Read the model definition and answer for the solid it produces. Units are mm, in the model's axes. A direction names the side the tool comes from. Coordinates: 2 decimals unless noted, no trailing zeros. Loops run counter-clockwise (first coordinate to the right, second up) from the corner with the lowest first, then second, coordinate; pieces in that order, holes last. Notation, with made-up numbers: (13, 88.5) -> (26, 88.5) arc R13 cw to (26, 94.5) -> close; hole circle Ø9 at (-17.75, -12). An arc over 180 degrees is marked (long way). Answer in a Markdown table with one row per item.
```python
from build123d import *

# Parameters (mm, degrees)
BOSS_EXTRUDE1_DEPTH = 24
SKETCH2_R           = 5
BOSS_EXTRUDE2_DEPTH = 16
FILLET1_R           = 2
SKETCH4_W           = 5.41
SKETCH4_H           = 3.8
CUT_EXTRUDE1_DEPTH  = 20


with BuildPart() as part:
    # Sketch1 → Boss-Extrude1 (new body)
    with BuildSketch(Plane(origin=(0, 0, 0), x_dir=(0, 0, -1), z_dir=(1, 0, 0))):
        with BuildLine():
            Line((2.314035395, 32.242240005), (10.473918124, 39.089194593))
            Line((10.473918124, 39.089194593), (14.117106565, 29.079616616))
            ThreePointArc((14.117106565, 29.079616616), (15.7, 27.193197679), (18.12513344, 26.765581222))
            Line((18.12513344, 26.765581222), (28.615276469, 28.615276469))
            Line((28.615276469, 28.615276469), (26.765581222, 18.12513344))
            ThreePointArc((26.765581222, 18.12513344), (27.193197679, 15.7), (29.079616616, 14.117106565))
            Line((29.079616616, 14.117106565), (39.089194593, 10.473918124))
            Line((39.089194593, 10.473918124), (32.242240005, 2.314035395))
            ThreePointArc((32.242240005, 2.314035395), (31.4, 0), (32.242240005, -2.314035395))
            Line((32.242240005, -2.314035395), (39.089194593, -10.473918124))
            Line((39.089194593, -10.473918124), (29.079616616, -14.117106565))
            ThreePointArc((29.079616616, -14.117106565), (27.193197679, -15.7), (26.765581222, -18.12513344))
            Line((26.765581222, -18.12513344), (28.615276469, -28.615276469))
            Line((28.615276469, -28.615276469), (18.12513344, -26.765581222))
            ThreePointArc((18.12513344, -26.765581222), (15.7, -27.193197679), (14.117106565, -29.079616616))
            Line((14.117106565, -29.079616616), (10.473918124, -39.089194593))
            Line((10.473918124, -39.089194593), (2.314035395, -32.242240005))
            ThreePointArc((2.314035395, -32.242240005), (0, -31.4), (-2.314035395, -32.242240005))
            Line((-2.314035395, -32.242240005), (-10.473918124, -39.089194593))
            Line((-10.473918124, -39.089194593), (-14.117106565, -29.079616616))
            ThreePointArc((-14.117106565, -29.079616616), (-15.7, -27.193197679), (-18.12513344, -26.765581222))
            Line((-18.12513344, -26.765581222), (-28.615276469, -28.615276469))
            Line((-28.615276469, -28.615276469), (-26.765581222, -18.12513344))
            ThreePointArc((-26.765581222, -18.12513344), (-27.193197679, -15.7), (-29.079616616, -14.117106565))
            Line((-29.079616616, -14.117106565), (-39.089194593, -10.473918124))
            Line((-39.089194593, -10.473918124), (-32.242240005, -2.314035395))
            ThreePointArc((-32.242240005, -2.314035395), (-31.4, 0), (-32.242240005, 2.314035395))
            Line((-32.242240005, 2.314035395), (-39.089194593, 10.473918124))
            Line((-39.089194593, 10.473918124), (-29.079616616, 14.117106565))
            ThreePointArc((-29.079616616, 14.117106565), (-27.193197679, 15.7), (-26.765581222, 18.12513344))
            Line((-26.765581222, 18.12513344), (-28.615276469, 28.615276469))
            Line((-28.615276469, 28.615276469), (-18.12513344, 26.765581222))
            ThreePointArc((-18.12513344, 26.765581222), (-15.7, 27.193197679), (-14.117106565, 29.079616616))
            Line((-14.117106565, 29.079616616), (-10.473918124, 39.089194593))
            Line((-10.473918124, 39.089194593), (-2.314035395, 32.242240005))
            ThreePointArc((-2.314035395, 32.242240005), (0, 31.4), (2.314035395, 32.242240005))
        make_face()
    extrude(amount=BOSS_EXTRUDE1_DEPTH)

    # Sketch2 → Boss-Extrude2 (add)
    with BuildSketch(Plane(origin=(24, 0, 0), x_dir=(0, 0, -1), z_dir=(1, 0, 0))):
        Circle(SKETCH2_R)
    extrude(amount=BOSS_EXTRUDE2_DEPTH)

    # Fillet1
    fillet1_edges = [part.edges().sort_by_distance(p)[0] for p in [
        (24, 0, 5),
    ]]
    fillet(fillet1_edges, radius=FILLET1_R)

    # Sketch4 → Cut-Extrude1 (cut)
    with BuildSketch(Plane(origin=(40, 0, 0), x_dir=(0, 0, -1), z_dir=(1, 0, 0))):
        Rectangle(SKETCH4_W, SKETCH4_H)
    extrude(amount=-CUT_EXTRUDE1_DEPTH, mode=Mode.SUBTRACT)


solid = part.part
```
1. Given pin 1 Ø1.9 at (x, y) = (26, -1) entering from +Z; pin 2 Ø3 at (x, y) = (9.5, -4.5) entering from -Z; pin 3 Ø1.1 at (x, y) = (34.5, -1) entering from -Z; pin 4 Ø5 at (y, z) = (-17.5, -30) entering from -X, each flat-ended and moving along its own axis, determine where each tip first touches the part or whether it passes through.
A:
| item | result |
|---|---|
| pin 1 | stops at z = 5.17 |
| pin 2 | stops at z = -35.34 |
| pin 3 | stops at z = -4.98 |
| pin 4 | passes through |
2. The mould has two halves that part along Z. Classify faces 5 (the flat face through (11.832, 6.451, -35.714)), 6 (the cylindrical face through (11.832, -27.176, -15.731)), 7 (the flat face through (11.832, -23.444, 27.703)): pulls with the +Z half, pulls with the -Z half, needs draft (parallel to the pull), parting line crosses it, or undercut.
A:
| item | result |
|---|---|
| face 5 | pulls with the -Z half |
| face 6 | undercut |
| face 7 | pulls with the +Z half |
3. A tool of negligible diameter and unlimited length cuts with its end or side. For faces 1 (the flat face through (11.832, 27.703, 23.444)), 2 (the flat face through (20, 0, 0)), 3 (the flat face through (11.83, 23.3, 27.68)), 4 (the flat face through (11.83, -23.3, -27.68)), from which of +Z, -Z, +X, -X, +Y, -Y can it reach the whole face along a straight path? Write none if from no direction.
A:
| item | result |
|---|---|
| face 1 | +X, -X, +Y |
| face 2 | +X |
| face 3 | +Z, +X, -X |
| face 4 | -Z, +X, -X |
4. Find the intervals of material crossed by probe 1 along X at (y, z) = (-1.5, 1); probe 2 along X at (y, z) = (-32, -3); probe 3 along Y at (x, z) = (23, 17), in increasing order.
A:
| item | result |
|---|---|
| probe 1 | x = 0 to 20 |
| probe 2 | x = 0 to 24 |
| probe 3 | y = -26.75 to 26.75 |
5. A cutting plane is placed at A-A on y = 0. Give the vertices of the cut face in (x, z) (3 decimals), and give its area (3 significant figures).
A:
| item | result |
|---|---|
| outline | (0, -31.4) -> (24, -31.4) -> (24, -7) arc R2 cw to (26, -5) -> (40, -5) -> (40, -2.705) -> (20, -2.705) -> (20, 2.705) -> (40, 2.705) -> (40, 5) -> (26, 5) arc R2 cw to (24, 7) -> (24, 31.4) -> (0, 31.4) -> close |
| area | 1,560 mm2 |
6. A cutting plane is placed at B-B on z = 0. Give the vertices of the cut face in (x, y), and give its area (3 significant figures).
A:
| item | result |
|---|---|
| outline | (0, -31.4) -> (24, -31.4) -> (24, -7) arc R2 cw to (26, -5) -> (40, -5) -> (40, -1.9) -> (20, -1.9) -> (20, 1.9) -> (40, 1.9) -> (40, 5) -> (26, 5) arc R2 cw to (24, 7) -> (24, 31.4) -> (0, 31.4) -> close |
| area | 1,590 mm2 |
7. A cutting plane is placed at C-C on x = 34. Give the vertices of the cut face in (y, z) (3 decimals), and give its area (3 significant figures).
A:
| item | result |
|---|---|
| outline | circle Ø10 at (0, 0); hole (-1.9, -2.705) -> (1.9, -2.705) -> (1.9, 2.705) -> (-1.9, 2.705) -> close |
| area | 58.0 mm2 |
8. A cutting plane is placed at D-D on z = 13. Give the vertices of the cut face in (x, y).
A:
| item | result |
|---|---|
| outline | (0, -32.15) -> (24, -32.15) -> (24, 32.15) -> (0, 32.15) -> close |
